```python
from build123d import *

# Parameters (mm, degrees)
SKETCH1_W           = 14
SKETCH1_H           = 10.5
BOSS_EXTRUDE1_DEPTH = 5
HOLE1_D             = 2.2
HOLE1_CBORE_D       = 4.2
HOLE1_CBORE_DEPTH   = 1.3
FILLET_2_R          = 3
M2X0_4_5_D          = 1.6


with BuildPart() as part:
    # Sketch1 → Boss-Extrude1 (new body)
    with BuildSketch(Plane(origin=(0, 0, 0), x_dir=(1, 0, 0), z_dir=(0, 1, 0))):
        Rectangle(SKETCH1_W, SKETCH1_H)
    extrude(amount=BOSS_EXTRUDE1_DEPTH)

    # Hole1 (through all)
    with Locations(Plane.XZ):
        with Locations((-2, -2.05), (4, -2.05)):
            CounterBoreHole(HOLE1_D / 2, HOLE1_CBORE_D / 2, HOLE1_CBORE_DEPTH)

    # ﾌｨﾚｯﾄ2
    fillet_2_edges = [part.edges().sort_by_distance(p)[0] for p in [
        (7, 2.5, 5.25),
    ]]
    fillet(fillet_2_edges, radius=FILLET_2_R)

    # M2x0.4 ねじ穴5 (through all)
    with Locations(Plane(origin=(-5, 2.5, 5.25), x_dir=(1, 0, 0), z_dir=(0, 0, 1))):
        with Locations((0, 0), (6, 0)):
            Hole(M2X0_4_5_D / 2)


solid = part.part
```
Check sheet for the modelled part. Datum: model origin and axes. Units: mm. A direction names the side the tool comes from. Give positions to 0.01 mm unless a question says otherwise; leave off trailing zeros. Loops run counter-clockwise (first coordinate to the right, second up) from the corner with the lowest first, then second, coordinate; pieces in that order, holes last. Notation, with made-up numbers: M 50.25,-14.75 L 89.25,-14.75 A23 ccw 89.25,8.25 Z; hole C 76.5,-3.5 d1. An arc over 180 degrees is marked long. Answer in a Markdown table with one row per item.
1) Cross-section at B-B (z = -2.05). Enter the section's corners in (x, y).
Solutions:
| item | result |
|---|---|
| outline | M -7,0 L -4.1,0 L -4.1,1.3 L -3.1,1.3 L -3.1,5 L -7,5 Z; M -0.9,1.3 L 0.1,1.3 L 0.1,0 L 1.9,0 L 1.9,1.3 L 2.9,1.3 L 2.9,5 L -0.9,5 Z; M 5.1,1.3 L 6.1,1.3 L 6.1,0 L 7,0 L 7,5 L 5.1,5 Z; hole C -5,2.5 d1.6; hole C 1,2.5 d1.6 |
2) Cross-section at A-A (x = -2). Enter the section's corners in (y, z), plus the area to 3 significant figures.
Solutions:
| item | result |
|---|---|
| outline | M 0,-5.25 L 5,-5.25 L 5,-3.15 L 1.3,-3.15 L 1.3,-4.15 L 0,-4.15 Z; M 0,0.05 L 1.3,0.05 L 1.3,-0.95 L 5,-0.95 L 5,5.25 L 0,5.25 Z |
| area | 38.9 mm^2 |
3) Mould release check, pull along X, two halves, no side actions. Record for faces 3 (the face through (-3.05, 3.18, -1.72)), 4 (the face through (7, 2, -1)), 5 (the face through (-2, 2, 5.25)): released by +X, released by -X, zero draft, split by the parting line, or undercut.
Solutions:
| item | result |
|---|---|
| face 3 | undercut |
| face 4 | released by +X |
| face 5 | zero draft |
4) Depth check by flat-ended pin: pin 1 (1.4 mm diameter, centred on x = 1, y = 2.5, fed in from +Z); pin 2 (2.5 mm diameter, centred on x = 4, z = -2.05, fed in from -Y). Enter the tip coordinate at first touch or a pass-through.
Solutions:
| item | result |
|---|---|
| pin 1 | passes through |
| pin 2 | stops at y = 1.3 |
5) Thickness scan on line 1 (X direction, y = 2.55, z = 0.5); line 2 (Z direction, x = -2, y = 0.95); line 3 (Z direction, x = 4, y = 3.8). Record the ranges inside material, lowest first.
Solutions:
| item | result |
|---|---|
| line 1 | x = -7 to -5.8, -4.2 to 0.2, 1.8 to 7 |
| line 2 | z = -5.25 to -4.15, 0.05 to 5.25 |
| line 3 | z = -5.25 to -3.15, -0.95 to 5.25 |
6) Tool access check on faces 1 (the face through (-1.031, 0.641, -3.913)), 2 (the face through (2.95, 3.18, -1.72)). Record the directions out of +Z, -Z, +X, -X, +Y, -Y that give a thin tool (end or side, any length) a straight path to the whole face; none if there is none.
Solutions:
| item | result |
|---|---|
| face 1 | -Y |
| face 2 | +Y, -Y |
7) Cross-section at C-C (y = 3.55). Enter the section's corners in (x, z), plus the area to 3 significant figures.
Solutions:
| item | result |
|---|---|
| outline | M -7,-5.25 L 7,-5.25 L 7,2.25 A3 ccw 4,5.25 L -7,5.25 Z; hole C -2,-2.05 d2.2; hole C 4,-2.05 d2.2 |
| area | 137 mm^2 |
8) Cross-section at D-D (y = 2.5). Enter the section's corners in (x, z), plus the area to 3 significant figures.
Solutions:
| item | result |
|---|---|
| outline | M -7,-5.25 L -5.8,-5.25 L -5.8,5.25 L -7,5.25 Z; M -4.2,-5.25 L 0.2,-5.25 L 0.2,5.25 L -4.2,5.25 Z; M 1.8,-5.25 L 7,-5.25 L 7,2.25 A3 ccw 4,5.25 L 1.8,5.25 Z; hole C -2,-2.05 d2.2; hole C 4,-2.05 d2.2 |
| area | 104 mm^2 |
